Geometry: final body of the model. Coordinates: model frame, mm. Coordinates: 2 decimals unless noted, no trailing zeros. Answer as a JSON object with one key per item and string values. Group by question number.
Item 1: Mould query, pull axis Y, two halves, no side actions, for faces 1 (the cylindrical face through (-825.9, -6, 356.6)), 2 (the flat face through (-814.016, 5.861, 353.301)), 3 (the flat face through (-821.43, -5.94, 350.01)), 4 (the flat face through (-823.175, -5.473, 349.15)). Classes: pulls with the +Y half, pulls with the -Y half, needs draft (parallel to the pull), parting line crosses it, or undercut.
Item 2: First-contact query: pin 1 Ø4 at (x, y) = (-820.5, -5.5) entering from -Z; pin 2 Ø2 at (x, z) = (-813.5, 356.5) entering from +Y; pin 3 Ø12 at (x, z) = (-812.5, 360.5) entering from +Y. Flat tips, straight axial feed; report the tip coordinate or a pass-through.
Item 3: Line query: line 1 along Y through (x, z) = (-821.5, 353.5); line 2 along Z through (x, y) = (-823.25, 0.5); line 3 along Z through (x, y) = (-814.25, 8). Output: solid intervals per line, ascending. Write a range as from..to.
```python
from build123d import *

# Parameters (mm, degrees)
SKETCH_1_R      = 1.5
SKETCH_1_R_2    = 6.5
EXTRUDE_1_DEPTH = 5
SKETCH_3_R      = 8
EXTRUDE_2_DEPTH = 2


with BuildPart() as part:
    # Эскиз1 → Бобышка-Вытянуть1 (new body)
    with BuildSketch(Plane(origin=(-480.803789864, 134.652080906, -243.886731474), x_dir=(0.4444744759103933, -0.03421577425644369, -0.8951378223805614), z_dir=(0.865247481188387, -0.24231791906874578, 0.4388950015611307))):
        with BuildLine():
            Line((-688.122906945, -142.837632594), (-688.122906945, -168.837632594))
            ThreePointArc((-688.122906945, -168.837632594), (-678.122906945, -178.837632594), (-668.122906945, -168.837632594))
            Line((-668.122906945, -168.837632594), (-668.122906945, -142.837632594))
            ThreePointArc((-668.122906945, -142.837632594), (-678.122906945, -132.837632594), (-688.122906945, -142.837632594))
        make_face()
        with Locations(Location((-678.122906945, -142.837632594, 0), (0, 0, 2.021059913))):
            Circle(SKETCH_1_R, mode=Mode.SUBTRACT)
        with Locations(Location((-678.122906945, -168.837632594, 0), (0, 0, 2.021059913))):
            Circle(SKETCH_1_R_2, mode=Mode.SUBTRACT)
    extrude(amount=EXTRUDE_1_DEPTH)

    # Эскиз3 → Бобышка-Вытянуть2 (add)
    with BuildSketch(Plane(origin=(-480.803789864, 134.652080906, -243.886731474), x_dir=(0.10581409215127123, 0.9439807153609489, 0.31257604983241044), z_dir=(-0.865247481188387, 0.24231791906874575, -0.4388950015611306))):
        with Locations(Location((16.948979253, -698.619750083, 0), (0, 0, 103.349815393))):
            Circle(SKETCH_3_R)
    extrude(amount=EXTRUDE_2_DEPTH)


solid = part.part
```
Checks:
{
 "1": {"face 1": "undercut", "face 2": "pulls with the -Y half", "face 3": "undercut", "face 4": "pulls with the +Y half"},
 "2": {"pin 1": "z = 341.87", "pin 2": "y = 28.6", "pin 3": "y = 28.89"},
 "3": {"line 1": "-15.98..-12.03, -0.41..1.32", "line 2": "352.6..354.57, 357.15..359.94", "line 3": "343.55..354.94"}
}
